Study the drawing (mm; zero at the part's minimum x, y, z) and answer. A direction names the side the tool comes from. Coordinates: 2 decimals unless noted, no trailing zeros. Write each loop counter-clockwise with the first axis right and the second up, starting at its lowest first coordinate (ties: lowest second). Pieces come first, ordered by that corner, then holes. Notation, with made-up numbers: (-32, -39) - (12, -39) arc R21 ccw to (12, -8) - close; hole circle Ø2 at (52, 47.25). An arc over 180 degrees is marked (long way). One line per item, written item: value.
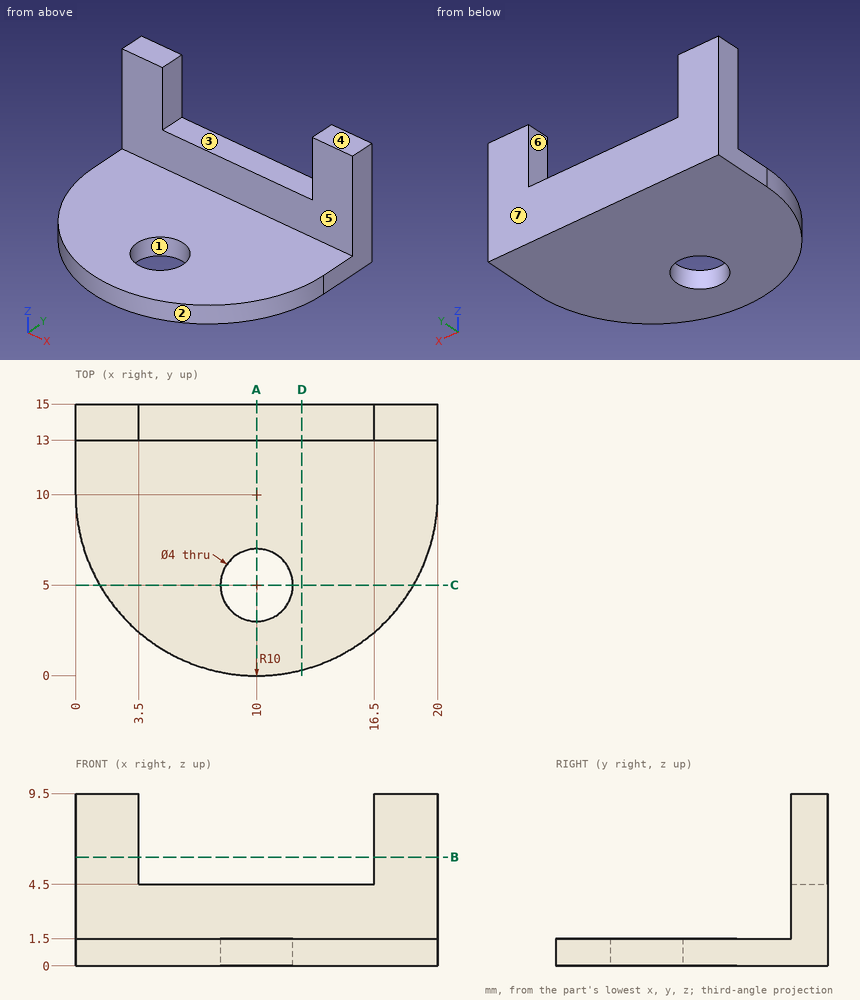
Item 1: Determine the mould class of the marked faces 1, 2, 3 and 4 for opening direction X: +X half, -X half, draft (parallel to the pull), parting line (faces both ways), or undercut.
Evaluation:
face 1: undercut
face 2: parting line
face 3: undercut
face 4: draft
Item 2: Given pin 1 (6.5 mm diameter, centred on x = 6, y = 4, fed in from +Z); pin 2 (1.6 mm diameter, centred on x = 7.5, y = 14.5, fed in from +Z); pin 3 (2 mm diameter, centred on x = 9.5, z = 5, fed in from -Y); pin 4 (2.5 mm diameter, centred on x = 10, y = 5, fed in from -Z), each flat-ended and moving along its own axis, determine where each tip first touches the part or whether it passes through.
Evaluation:
pin 1: stops at z = 1.5
pin 2: stops at z = 4.5
pin 3: stops at y = 13
pin 4: passes through
Item 3: Section B-B, the plane z = 6 is taken. Determine the outline of the cut face in (x, y).
Evaluation:
outline: (0, 13) - (3.5, 13) - (3.5, 15) - (0, 15) - close; (16.5, 13) - (20, 13) - (20, 15) - (16.5, 15) - close
Item 4: Section D-D, the plane x = 12.5 is taken. Determine the outline of the cut face in (y, z).
Evaluation:
outline: (0.32, 0) - (15, 0) - (15, 4.5) - (13, 4.5) - (13, 1.5) - (0.32, 1.5) - close
Item 5: Section C-C, the plane y = 5 is taken. Determine the outline of the cut face in (x, z).
Evaluation:
outline: (1.34, 0) - (8, 0) - (8, 1.5) - (1.34, 1.5) - close; (12, 0) - (18.66, 0) - (18.66, 1.5) - (12, 1.5) - close
Item 6: Which of the six approach directions +Z, -Z, +X, -X, +Y, -Y give full straight-line access (tool end or side, diameter ignored) to the marked faces 5, 6 and 7?
Evaluation:
face 5: +Z, +X, -X, -Y
face 6: +Z, +Y, -Y
face 7: +Z, -Z, +X, -X, +Y
Item 7: Section A-A, the plane x = 10 is taken. Determine the outline of the cut face in (y, z).
Evaluation:
outline: (0, 0) - (3, 0) - (3, 1.5) - (0, 1.5) - close; (7, 0) - (15, 0) - (15, 4.5) - (13, 4.5) - (13, 1.5) - (7, 1.5) - close
Item 8: Consider probe 1 along X at (y, z) = (13.5, 5.5); probe 2 along Y at (x, z) = (10, 0.45); probe 3 along Z at (x, y) = (19, 8.25). Determine where each line is inside the solid, lowest interval first.
Evaluation:
probe 1: x = 0 to 3.5, 16.5 to 20
probe 2: y = 0 to 3, 7 to 15
probe 3: z = 0 to 1.5
